Work out the finished part from the listing and answer in its coordinate system (mm). A direction names the side the tool comes from. Coordinates: 2 decimals unless noted, no trailing zeros. Loops run counter-clockwise (first coordinate to the right, second up) from the corner with the lowest first, then second, coordinate; pieces in that order, holes last. Notation, with made-up numbers: (18, 10.25) -> (54, 10.25) arc R24 ccw to (54, 34.25) -> close; hole circle Ø3 at (-1, 36.5). An arc over 180 degrees is marked (long way). Use a Markdown table: item, result.
from build123d import *

# Parameters (mm, degrees)
BOSS_EXTRUDE1_DEPTH = 64
CUT_EXTRUDE1_DEPTH  = 4


with BuildPart() as part:
    # Sketch1 → Boss-Extrude1 (new body)
    with BuildSketch(Plane.XY):
        Polygon((0, 0), (7.5, 0), (41.081225522, 52.711965363), (39.456184018, 61.933802982), align=None)
    extrude(amount=BOSS_EXTRUDE1_DEPTH)

    # Sketch2 → Cut-Extrude1 (cut)
    with BuildSketch(Plane(origin=(48.852955135, 8.608705004, 0), x_dir=(0, 0, -1), z_dir=(0.9848263256181995, 0.1735428142256437, 0))):
        Polygon((-32, 44.782779676), (-28, 44.782779676), (-28, 47.782779676), (-36, 47.782779676), (-36, 44.782779676), align=None)
    extrude(amount=-CUT_EXTRUDE1_DEPTH, mode=Mode.SUBTRACT)


solid = part.part
Q1. Consider line 1 (Y direction, x = 22.5, z = 5); line 2 (X direction, y = 22.5, z = 23); line 3 (X direction, y = 59.5, z = 17). Determine where each line is inside the solid, lowest interval first. Write a range as [from, to].
Solved:
| item | result |
|---|---|
| line 1 | [23.55, 35.32] |
| line 2 | [14.33, 21.83] |
| line 3 | [37.91, 39.89] |
Q2. Given pin 1 Ø2 at (x, z) = (16, 21.5) entering from -Y; pin 2 Ø2 at (y, z) = (17.5, 20) entering from -X; pin 3 Ø12 at (x, y) = (32, 24) entering from -Z; pin 4 Ø5 at (x, z) = (21.5, 50.5) entering from -Y, each flat-ended and moving along its own axis, determine where each tip first touches the part or whether it passes through.
Solved:
| item | result |
|---|---|
| pin 1 | y = 11.77 |
| pin 2 | x = 10.51 |
| pin 3 | through |
| pin 4 | y = 18.05 |
Q3. Section B-B on x = 38 is taken. Determine the outline of the cut face in (y, z), and give its area (3 significant figures).
Solved:
| item | result |
|---|---|
| outline | (47.88, 0) -> (59.65, 0) -> (59.65, 64) -> (47.88, 64) -> close; hole (52.17, 28) -> (55.22, 28) -> (55.22, 36) -> (52.17, 36) -> close |
| area | 729 mm² |
Q4. Section D-D on x = 4.5 is taken. Determine the outline of the cut face in (y, z), and give its area (3 significant figures).
Solved:
| item | result |
|---|---|
| outline | (0, 0) -> (7.06, 0) -> (7.06, 64) -> (0, 64) -> close |
| area | 452 mm² |
Q5. Section A-A on z = 29.5 is taken. Determine the outline of the cut face in (x, y), and give its area (3 significant figures).
Solved:
| item | result |
|---|---|
| outline | (0, 0) -> (7.5, 0) -> (41.08, 52.71) -> (37.14, 52.02) -> (36.62, 54.97) -> (40.56, 55.67) -> (39.46, 61.93) -> close |
| area | 418 mm² |
Q6. For faces 1 (the flat face through (22, 29, 0)), 2 (the flat face through (36.878, 53.516, 32.056)), determine the directions among +Z, -Z, +X, -X, +Y, -Y from which every point of the face is accessible in a straight line to the end or side of a thin tool.
Solved:
| item | result |
|---|---|
| face 1 | -Z, +X, -X, +Y, -Y |
| face 2 | none |
Q7. Determine the mould class of faces 3 (the flat face through (38.619, 55.324, 31.944)), 4 (the flat face through (22, 29, 64)), 5 (the flat face through (20.004, 31.4, 31.552)), 6 (the flat face through (24.056, 25.987, 31.552)) for opening direction Y: pulls with the +Y half, pulls with the -Y half, needs draft (parallel to the pull), parting line crosses it, or undercut.
Solved:
| item | result |
|---|---|
| face 3 | undercut |
| face 4 | needs draft |
| face 5 | pulls with the +Y half |
| face 6 | pulls with the -Y half |
Q8. Section C-C on y = 58 is taken. Determine the outline of the cut face in (x, z).
Solved:
| item | result |
|---|---|
| outline | (36.95, 0) -> (40.15, 0) -> (40.15, 64) -> (36.95, 64) -> close |
